Can you work these out from the model? Positions are in its coordinate system, mm. A direction names the side the tool comes from. Round coordinates to 2 decimals unless told otherwise and drop trailing zeros. Loops run counter-clockwise (first coordinate to the right, second up) from the corner with the lowest first, then second, coordinate; pieces in that order, holes last.
(1) Which directions (+Z, -Z, +X, -X, +Y, -Y) give clear straight access to the entire face, cutting with the end or side of a thin tool? Please do faces 1 (the face through (3, 25.4, -49)), 2 (the face through (3, 33.338, -60)), 3 (the face through (3, 0, 6)).
(2) If I drill on line 1 along Z through (x, y) = (3.5, 29.5); line 2 along Z through (x, y) = (5.75, 33); line 3 along Z through (x, y) = (4.5, 16.5), over which ranges is the centre line in solid material (lowest first)?
(3) I want a section at D-D on y = 9. Write out the boundary of the cut face in (x, z), plus the area to 3 significant figures.
(4) I want a section at C-C on z = -37.5. Write out the boundary of the cut face in (x, y).
(5) Thinking about a two-plate mould opening in Z: for faces 4 (the face through (3.131, 16.501, -34.637)), 5 (the face through (3.131, 17.651, -14.137)), 6 (the face through (3.13, 29.82, -48)), which applies, released by +Z, released by -Z, zero draft, split by the parting line, or undercut?
(6) Will these pins go through, and if not, where does the flat tip stop? pin 1 Ø5 at (y, z) = (31.75, -50.52) entering from -X; pin 2 Ø2.5 at (x, z) = (3, -49.5) entering from -Y; pin 3 Ø8 at (y, z) = (25, -24) entering from +X; pin 4 Ø1.5 at (x, y) = (4.5, 26) entering from -Z.
(7) I want a section at B-B on y = 31.75. Write out the boundary of the cut face in (x, z).
from build123d import *

# Parameters (mm, degrees)
SKETCH2_R           = 3.175
BOSS_EXTRUDE1_DEPTH = 6.35
FILLET1_R           = 40.64


with BuildPart() as part:
    # Sketch2 → Boss-Extrude1 (new body)
    # profile 1 of 2: a face of its own
    with BuildSketch(Plane(origin=(0, 0, 0), x_dir=(0, 0, -1), z_dir=(1, 0, 0))):
        with BuildLine():
            ThreePointArc((40.061425782, 35.803230962), (43.52688287, 37.512205275), (47.345846523, 38.1))
            Line((47.345846523, 38.1), (50.520846523, 38.1))
            ThreePointArc((50.520846523, 38.1), (56.870846523, 31.75), (50.520846523, 25.4))
            Line((50.520846523, 25.4), (47.345846523, 25.4))
            Line((47.345846523, 25.4), (11.070887152, 0))
            Line((11.070887152, 0), (-11.070887152, 0))
            Line((-11.070887152, 0), (40.061425782, 35.803230962))
        make_face()
        with Locations((50.520846523, 31.75)):
            Circle(SKETCH2_R, mode=Mode.SUBTRACT)
    # profile 2 of 2: a face of its own
    with BuildSketch(Plane(origin=(0, 0, 0), x_dir=(0, 0, -1), z_dir=(1, 0, 0))):
        with BuildLine():
            ThreePointArc((56.669207586, 33.3375), (56.870846523, 31.75), (56.669207586, 30.1625))
            Line((56.669207586, 30.1625), (63.220846523, 30.1625))
            Line((63.220846523, 30.1625), (63.220846523, 33.3375))
            Line((63.220846523, 33.3375), (56.669207586, 33.3375))
        make_face()
    extrude(amount=BOSS_EXTRUDE1_DEPTH)

    # Fillet1
    fillet1_edges = [part.edges().sort_by_distance(p)[0] for p in [
        (3.175, 0, -11.070887152),
    ]]
    fillet(fillet1_edges, radius=FILLET1_R)


solid = part.part
Filled sheet:
1. face 1: -Z, +X, -X, -Y
1. face 2: -Z, +X, -X, +Y
1. face 3: +Z, -Z, +X, -X, -Y
2. line 1: z = -56.46 to -52.76, -48.28 to -31.06
2. line 2: z = -63.22 to -53.44, -47.6 to -36.06
2. line 3: z = -34.64 to -12.49
3. outline: (0, -23.92) - (6.35, -23.92) - (6.35, -1.78) - (0, -1.78) - close
3. area: 141 mm2
4. outline: (0, 18.51) - (6.35, 18.51) - (6.35, 34.01) - (0, 34.01) - close
5. face 4: released by -Z
5. face 5: released by +Z
5. face 6: undercut
6. pin 1: passes through
6. pin 2: stops at y = 25.4
6. pin 3: stops at x = 6.35
6. pin 4: stops at z = -54.44
7. outline: (0, -63.22) - (6.35, -63.22) - (6.35, -53.7) - (0, -53.7) - close; (0, -47.35) - (6.35, -47.35) - (6.35, -34.27) - (0, -34.27) - close
